Can you work these out from the drawing? Everything is in mm from the part's minimum corner. Round coordinates to 2 decimals unless told otherwise and drop trailing zeros. Loops run counter-clockwise (first coordinate to the right, second up) from the corner with the lowest first, then second, coordinate; pieces in that order, holes last. Notation, with made-up numbers: M -7.75,29.5 L 6.25,29.5 A14 ccw 6.25,36.5 Z; hole C -7,24.25 d3. An arc over 180 degrees is marked long. Answer in a Markdown table with one row per item.
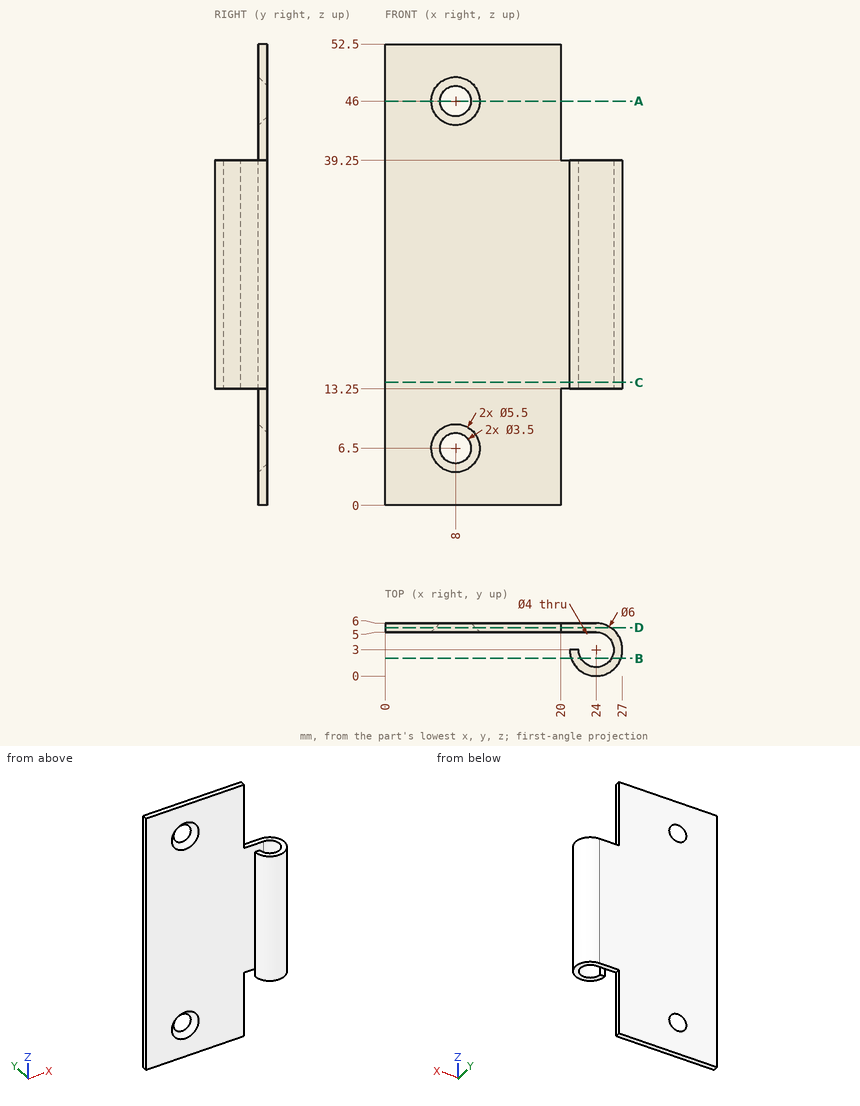
1) I want a section at A-A, the plane z = 46. Please give me the cut outline in (x, y), plus the area to 3 significant figures.
Computed:
| item | result |
|---|---|
| outline | M 0,5 L 5.25,5 L 6.25,6 L 0,6 Z; M 9.75,6 L 10.75,5 L 20,5 L 20,6 Z |
| area | 15.5 mm² |
2) I need wall thicknesses on line 1 (Y direction, x = 24, z = 29.5); line 2 (Y direction, x = 3.75, z = 47.5); line 3 (X direction, y = 1.5, z = 21.5). Which ranges of each line are inside material? Lowest first, please.
Computed:
| item | result |
|---|---|
| line 1 | y = 0 to 1, 5 to 6 |
| line 2 | y = 5 to 6 |
| line 3 | x = 21.4 to 22.68, 25.32 to 26.6 |
3) I want a section at B-B, the plane y = 2. Please give me the cut outline in (x, z), plus the area to 3 significant figures.
Computed:
| item | result |
|---|---|
| outline | M 21.17,13.25 L 22.27,13.25 L 22.27,39.25 L 21.17,39.25 Z; M 25.73,13.25 L 26.83,13.25 L 26.83,39.25 L 25.73,39.25 Z |
| area | 57.0 mm² |
4) I want a section at C-C, the plane z = 14. Please give me the cut outline in (x, y), plus the area to 3 significant figures.
Computed:
| item | result |
|---|---|
| outline | M 0,5 L 24,5 A2 cw long 22,3 L 21,3 A3 ccw long 24,6 L 0,6 Z |
| area | 35.8 mm² |
5) Will these pins go through, and if not, where does the flat tip stop? P1, Ø0.8, axis at y = 5.5, z = 5, coming from the +X side; P2, Ø7, axis at x = 15, z = 31.5, coming from the -Y side; P3, Ø1.8, axis at x = 22.5, y = 1.5, coming from the -Z side.
Computed:
| item | result |
|---|---|
| P1 | stops at x = 20 |
| P2 | stops at y = 5 |
| P3 | stops at z = 13.25 |
6) I want a section at D-D, the plane y = 5.5. Please give me the cut outline in (x, z).
Computed:
| item | result |
|---|---|
| outline | M 0,0 L 20,0 L 20,13.25 L 25.66,13.25 L 25.66,39.25 L 20,39.25 L 20,52.5 L 0,52.5 Z; hole C 8,6.5 d4.5; hole C 8,46 d4.5 |
